Can you work these out from the model? Positions are in its coordinate system, mm. A direction names the side the tool comes from. Coordinates: 2 decimals unless noted, no trailing zeros. Order: outer loops, then holes, each group sorted by start corner. A loop starts at its lowest first (then second) coordinate and runs counter-clockwise, first axis right, second up. Notation, with made-up numbers: (-24, 59) -> (-20, 59) arc R21 cw to (-20, 81) -> close; hole circle Ø9 at (-15.75, 86.5). An arc over 180 degrees is marked (long way). Use a Markdown table: item, result. Add a question column.
1. Suppose I cut it at C-C, the plane x = -311. List the corners of the cut face in (y, z) for me.
2. If I drill on line 1 along X through (y, z) = (3.5, -10.5); line 2 along Y through (x, z) = (504, -38); line 3 along X through (y, z) = (-7, 4), over which ranges is the centre line in solid material (lowest first)? Write a range as from..to.
3. We'd pull the mould along X, two halves only. Please class faces 1 (the flat face through (-5, 0, 1)), 2 (the flat face through (-545.566, -42.947, 98.604)), 3 (the flat face through (-383.05, -12.42, 1.09)): pulls with the +X half, pulls with the -X half, needs draft (parallel to the pull), parting line crosses it, or undercut.
4. Suppose I cut it at A-A, the plane z = 0. List the corners of the cut face in (x, y) for me, then the cut area to 3 significant figures.
5. For faces 4 (the flat face through (-520, -40, 1)), 5 (the flat face through (-516, -32, 1)), 6 (the flat face through (-379.4, -19.6, 1.1)), which set-ups out of +Z, -Z, +X, -X, +Y, -Y let a thin tool reach every point of the face, with its end or its side?
6. For pin 1 Ø9 at (x, y) = (566, -34) entering from -Z; pin 2 Ø9 at (y, z) = (-34.5, -11.5) entering from -X; pin 3 Ø2.5 at (x, y) = (-219.5, 3.5) entering from +Z, each with a flat end and sliding along its axis, tell me the tip position at first contact or that it passes through.
7. Suppose I cut it at B-B, the plane y = -13.5. List the corners of the cut face in (x, z) for me.
```python
from build123d import *

# Parameters (mm, degrees)
SM_BASE_FLANGE_1_DEPTH             = 77.5
SKETCH_6_W                         = 155
SKETCH_6_H                         = 65
CUT_EXTRUDE_1_DEPTH                = 687.083267541
CUT_EXTRUDE_2_DEPTH                = 687.083267541
SM_EDGE_FLANGE_2_STRIP_CUT_DEPTH   = 265.155589796
SM_EDGE_FLANGE_2_STRIP_CUT_2_DEPTH = 265.155589796
SM_EDGE_FLANGE_2_STRIP_CUT_3_DEPTH = 265.155589796
SM_EDGE_FLANGE_2_STRIP_CUT_4_DEPTH = 265.155589796
SM_EDGE_FLANGE_2_DEPTH             = 265.155589796
SM_EDGE_FLANGE_2_BEND_DEPTH        = 265.155589796
SM_EDGE_FLANGE_2_BEND_2_DEPTH      = 265.155589796
SM_EDGE_FLANGE_2_BEND_3_DEPTH      = 265.155589796
FILLET_1_R                         = 10
FILLET_2_R                         = 20


# Sheet-metal steps are written as plain solids
with BuildPart() as part:
    # Sketch 1 → 基体-法兰1 (new, symmetric)
    with BuildSketch(Plane.XY):
        with BuildLine():
            Line((-680, -40), (-414.844410204, -40))
            ThreePointArc((-414.844410204, -40), (-410.207863825, -39.313472424), (-405.969207064, -37.312804709))
            Line((-405.969207064, -37.312804709), (-352.015396468, -1.343597645))
            ThreePointArc((-352.015396468, -1.343597645), (-349.896068088, -0.343263788), (-347.577794898, 0))
            Line((-347.577794898, 0), (347.577794898, 0))
            ThreePointArc((347.577794898, 0), (349.896068088, -0.343263788), (352.015396468, -1.343597645))
            Line((352.015396468, -1.343597645), (405.969207064, -37.312804709))
            ThreePointArc((405.969207064, -37.312804709), (410.207863825, -39.313472424), (414.844410204, -40))
            Line((414.844410204, -40), (680, -40))
            Line((680, -40), (680, -32))
            Line((680, -32), (414.844410204, -32))
            ThreePointArc((414.844410204, -32), (412.526137014, -31.656736212), (410.406808634, -30.656402355))
            Line((410.406808634, -30.656402355), (356.452998038, 5.312804709))
            ThreePointArc((356.452998038, 5.312804709), (352.214341277, 7.313472424), (347.577794898, 8))
            Line((347.577794898, 8), (-347.577794898, 8))
            ThreePointArc((-347.577794898, 8), (-352.214341277, 7.313472424), (-356.452998038, 5.312804709))
            Line((-356.452998038, 5.312804709), (-410.406808634, -30.656402355))
            ThreePointArc((-410.406808634, -30.656402355), (-412.526137014, -31.656736212), (-414.844410204, -32))
            Line((-414.844410204, -32), (-680, -32))
            Line((-680, -32), (-680, -40))
        make_face()
    extrude(amount=SM_BASE_FLANGE_1_DEPTH, both=True)

    # 草图6 → 切除-拉伸1 (cut, through all)
    with BuildSketch(Plane(origin=(0, 8, 0), x_dir=(1, 0, 0), z_dir=(0, 1, 0))):
        with Locations((-602.5, 0)):
            Rectangle(SKETCH_6_W, SKETCH_6_H)
        with Locations((602.5, 0)):
            Rectangle(SKETCH_6_W, SKETCH_6_H)
    extrude(amount=-CUT_EXTRUDE_1_DEPTH, mode=Mode.SUBTRACT)

    # 草图7 → 切除-拉伸2 (cut, through all)
    with BuildSketch(Plane(origin=(0, 8, 0), x_dir=(1, 0, 0), z_dir=(0, 1, 0))):
        with BuildLine():
            Line((-225, 16), (-215, 16))
            ThreePointArc((-215, 16), (-199, 0), (-215, -16))
            Line((-215, -16), (-225, -16))
            ThreePointArc((-225, -16), (-241, 0), (-225, 16))
        make_face()
        with BuildLine():
            Line((215, 16), (225, 16))
            ThreePointArc((225, 16), (241, 0), (225, -16))
            Line((225, -16), (215, -16))
            ThreePointArc((215, -16), (199, 0), (215, 16))
        make_face()
    extrude(amount=-CUT_EXTRUDE_2_DEPTH, mode=Mode.SUBTRACT)

    # 边线-法兰2 strip (across the edge) → 边线-法兰2 strip cut (cut)
    with BuildSketch(Plane(origin=(-680, -40, -77.5), x_dir=(0, -0.8660254037844416, 0.49999999999999495), z_dir=(1, 0, 0))):
        Polygon((-29.856406461, 35.712812921), (-5.856406461, -5.856406461), (1.07179677, -1.856406461), (-22.92820323, 39.712812921), align=None)
    extrude(amount=SM_EDGE_FLANGE_2_STRIP_CUT_DEPTH, mode=Mode.SUBTRACT)

    # 边线-法兰2 strip 2 (across the edge) → 边线-法兰2 strip cut 2 (cut)
    with BuildSketch(Plane(origin=(680, -40, 77.5), x_dir=(0, -0.8660254037844416, -0.49999999999999495), z_dir=(-1, 0, 0))):
        Polygon((-29.856406461, 35.712812921), (-5.856406461, -5.856406461), (1.07179677, -1.856406461), (-22.92820323, 39.712812921), align=None)
    extrude(amount=SM_EDGE_FLANGE_2_STRIP_CUT_2_DEPTH, mode=Mode.SUBTRACT)

    # 边线-法兰2 strip 3 (across the edge) → 边线-法兰2 strip cut 3 (cut)
    with BuildSketch(Plane(origin=(414.844410204, -40, -77.5), x_dir=(0, -0.8660254037844416, 0.49999999999999495), z_dir=(1, 0, 0))):
        Polygon((-29.856406461, 35.712812921), (-5.856406461, -5.856406461), (1.07179677, -1.856406461), (-22.92820323, 39.712812921), align=None)
    extrude(amount=SM_EDGE_FLANGE_2_STRIP_CUT_3_DEPTH, mode=Mode.SUBTRACT)

    # 边线-法兰2 strip 4 (across the edge) → 边线-法兰2 strip cut 4 (cut)
    with BuildSketch(Plane(origin=(-414.844410204, -40, 77.5), x_dir=(0, -0.8660254037844416, -0.49999999999999495), z_dir=(-1, 0, 0))):
        Polygon((-29.856406461, 35.712812921), (-5.856406461, -5.856406461), (1.07179677, -1.856406461), (-22.92820323, 39.712812921), align=None)
    extrude(amount=SM_EDGE_FLANGE_2_STRIP_CUT_4_DEPTH, mode=Mode.SUBTRACT)

    # 边线-法兰2 section (across the edge) → 边线-法兰2 (add)
    with BuildSketch(Plane(origin=(-680, -40, -77.5), x_dir=(0, -0.8660254037844416, 0.49999999999999495), z_dir=(1, 0, 0))):
        with BuildLine():
            Line((-8, 2.143593539), (-8, 37.856406461))
            Line((-8, 37.856406461), (0, 37.856406461))
            Line((0, 37.856406461), (0, 2.143593539))
            ThreePointArc((0, 2.143593539), (0.27259339, 0.073041179), (1.07179677, -1.856406461))
            Line((1.07179677, -1.856406461), (-5.856406461, -5.856406461))
            ThreePointArc((-5.856406461, -5.856406461), (-7.454813221, -1.997511182), (-8, 2.143593539))
        make_face()
    extrude(amount=SM_EDGE_FLANGE_2_DEPTH)

    # 边线-法兰2 section 2 (across the edge) → 边线-法兰2 bend (add)
    with BuildSketch(Plane(origin=(680, -40, 77.5), x_dir=(0, -0.8660254037844416, -0.49999999999999495), z_dir=(-1, 0, 0))):
        with BuildLine():
            Line((-8, 2.143593539), (-8, 37.856406461))
            Line((-8, 37.856406461), (0, 37.856406461))
            Line((0, 37.856406461), (0, 2.143593539))
            ThreePointArc((0, 2.143593539), (0.27259339, 0.073041179), (1.07179677, -1.856406461))
            Line((1.07179677, -1.856406461), (-5.856406461, -5.856406461))
            ThreePointArc((-5.856406461, -5.856406461), (-7.454813221, -1.997511182), (-8, 2.143593539))
        make_face()
    extrude(amount=SM_EDGE_FLANGE_2_BEND_DEPTH)

    # 边线-法兰2 section 3 (across the edge) → 边线-法兰2 bend 2 (add)
    with BuildSketch(Plane(origin=(414.844410204, -40, -77.5), x_dir=(0, -0.8660254037844416, 0.49999999999999495), z_dir=(1, 0, 0))):
        with BuildLine():
            Line((-8, 2.143593539), (-8, 37.856406461))
            Line((-8, 37.856406461), (0, 37.856406461))
            Line((0, 37.856406461), (0, 2.143593539))
            ThreePointArc((0, 2.143593539), (0.27259339, 0.073041179), (1.07179677, -1.856406461))
            Line((1.07179677, -1.856406461), (-5.856406461, -5.856406461))
            ThreePointArc((-5.856406461, -5.856406461), (-7.454813221, -1.997511182), (-8, 2.143593539))
        make_face()
    extrude(amount=SM_EDGE_FLANGE_2_BEND_2_DEPTH)

    # 边线-法兰2 section 4 (across the edge) → 边线-法兰2 bend 3 (add)
    with BuildSketch(Plane(origin=(-414.844410204, -40, 77.5), x_dir=(0, -0.8660254037844416, -0.49999999999999495), z_dir=(-1, 0, 0))):
        with BuildLine():
            Line((-8, 2.143593539), (-8, 37.856406461))
            Line((-8, 37.856406461), (0, 37.856406461))
            Line((0, 37.856406461), (0, 2.143593539))
            ThreePointArc((0, 2.143593539), (0.27259339, 0.073041179), (1.07179677, -1.856406461))
            Line((1.07179677, -1.856406461), (-5.856406461, -5.856406461))
            ThreePointArc((-5.856406461, -5.856406461), (-7.454813221, -1.997511182), (-8, 2.143593539))
        make_face()
    extrude(amount=SM_EDGE_FLANGE_2_BEND_3_DEPTH)

    # 圆角1
    fillet_1_edges = [part.edges().sort_by_distance(p)[0] for p in [
        (-680, -36, 32.5),
        (-680, -36, -32.5),
        (680, -36, -32.5),
        (680, -36, 32.5),
    ]]
    fillet(fillet_1_edges, radius=FILLET_1_R)

    # 圆角2
    fillet_2_edges = [part.edges().sort_by_distance(p)[0] for p in [
        (-680, -55.464101615, -112.284609691),
        (-414.844410204, -55.464101615, -112.284609691),
        (680, -55.464101615, 112.284609691),
        (414.844410204, -55.464101615, 112.284609691),
        (414.844410204, -55.464101615, -112.284609691),
        (680, -55.464101615, -112.284609691),
        (-414.844410204, -55.464101615, 112.284609691),
        (-680, -55.464101615, 112.284609691),
    ]]
    fillet(fillet_2_edges, radius=FILLET_2_R)


solid = part.part
```
Worked out:
| question | item | result |
|---|---|---|
| 1 | outline | (0, -77.5) -> (8, -77.5) -> (8, 77.5) -> (0, 77.5) -> close |
| 2 | line 1 | x = -359.17..-237.07, -202.93..202.93, 237.07..359.17 |
| 2 | line 2 | y = -40..-32 |
| 2 | line 3 | x = -374.92..-360.5, 360.5..374.92 |
| 3 | face 1 | undercut |
| 3 | face 2 | needs draft |
| 3 | face 3 | pulls with the -X half |
| 4 | outline | (-525, -40) -> (-414.84, -40) arc R16 ccw to (-405.97, -37.31) -> (-352.02, -1.34) arc R8 cw to (-347.58, 0) -> (-241, 0) -> (-241, 8) -> (-347.58, 8) arc R16 ccw to (-356.45, 5.31) -> (-410.41, -30.66) arc R8 cw to (-414.84, -32) -> (-525, -32) -> close; (-199, 0) -> (199, 0) -> (199, 8) -> (-199, 8) -> close; (241, 0) -> (347.58, 0) arc R8 cw to (352.02, -1.34) -> (405.97, -37.31) arc R16 ccw to (414.84, -40) -> (525, -40) -> (525, -32) -> (414.84, -32) arc R8 cw to (410.41, -30.66) -> (356.45, 5.31) arc R16 ccw to (347.58, 8) -> (241, 8) -> close |
| 4 | area | 7,920 mm² |
| 5 | face 4 | +X, -X, -Y |
| 5 | face 5 | +Z, -Z, -X, +Y |
| 5 | face 6 | +Z, -Z, -Y |
| 6 | pin 1 | stops at z = -90.9 |
| 6 | pin 2 | stops at x = -525 |
| 6 | pin 3 | stops at z = 77.5 |
| 7 | outline | (-384.67, -77.5) -> (-370.25, -77.5) -> (-370.25, 77.5) -> (-384.67, 77.5) -> close; (370.25, -77.5) -> (384.67, -77.5) -> (384.67, 77.5) -> (370.25, 77.5) -> close |
